```python
from build123d import *

# Parameters (mm, degrees)
SKETCH1_W                   = 77
SKETCH1_H                   = 24
BOSS_EXTRUDE1_DEPTH         = 6
CUT_EXTRUDE1_REACH          = 8
TAP_DRILL_FOR_M3_TAP1_D     = 2.5
TAP_DRILL_FOR_M3_TAP1_DEPTH = 10
TAP_DRILL_FOR_M3_TAP1_TIP   = 0.751075774
TAP_DRILL_FOR_M3_TAP2_D     = 2.5
TAP_DRILL_FOR_M3_TAP2_DEPTH = 10
TAP_DRILL_FOR_M3_TAP2_TIP   = 0.751075774
FILLET1_R                   = 1.5


with BuildPart() as part:
    # Sketch1 → Boss-Extrude1 (new body)
    with BuildSketch(Plane(origin=(0, 0, 0), x_dir=(1, 0, 0), z_dir=(0, 1, 0))):
        with Locations((38.5, 12)):
            Rectangle(SKETCH1_W, SKETCH1_H)
    extrude(amount=BOSS_EXTRUDE1_DEPTH)

    # Sketch2 → Cut-Extrude1 (cut, up to next)
    with BuildSketch(Plane(origin=(0, 6, 0), x_dir=(1, 0, 0), z_dir=(0, 1, 0)), mode=Mode.PRIVATE) as cut_extrude1_sk1:
        Polygon((0, 18), (7, 18), (17.082489299, 11.821127911), (7, 6), (0, 6), align=None)
    cut_extrude1_tool1 = extrude(cut_extrude1_sk1.sketch, amount=-CUT_EXTRUDE1_REACH, mode=Mode.PRIVATE) & part.part
    add(cut_extrude1_tool1.solids().sort_by_distance((6.372388, 6, -11.975038))[0], mode=Mode.SUBTRACT)
    # Sketch2 → Cut-Extrude1 (cut, up to next)
    with BuildSketch(Plane(origin=(0, 6, 0), x_dir=(1, 0, 0), z_dir=(0, 1, 0)), mode=Mode.PRIVATE) as cut_extrude1_sk2:
        Polygon((11.391702814, 20), (65.608297186, 20), (39.5, 4), (37.5, 4), align=None)
    cut_extrude1_tool2 = extrude(cut_extrude1_sk2.sketch, amount=-CUT_EXTRUDE1_REACH, mode=Mode.PRIVATE) & part.part
    add(cut_extrude1_tool2.solids().sort_by_distance((38.5, 6, -14.476924))[0], mode=Mode.SUBTRACT)
    # Sketch2 → Cut-Extrude1 (cut, up to next)
    with BuildSketch(Plane(origin=(0, 6, 0), x_dir=(1, 0, 0), z_dir=(0, 1, 0)), mode=Mode.PRIVATE) as cut_extrude1_sk3:
        Polygon((77, 18), (70, 18), (59.917510701, 11.821127911), (70, 6), (77, 6), align=None)
    cut_extrude1_tool3 = extrude(cut_extrude1_sk3.sketch, amount=-CUT_EXTRUDE1_REACH, mode=Mode.PRIVATE) & part.part
    add(cut_extrude1_tool3.solids().sort_by_distance((70.627612, 6, -11.975038))[0], mode=Mode.SUBTRACT)
    # Sketch2 → Cut-Extrude1 (cut, up to next)
    with BuildSketch(Plane(origin=(0, 6, 0), x_dir=(1, 0, 0), z_dir=(0, 1, 0)), mode=Mode.PRIVATE) as cut_extrude1_sk4:
        Polygon((20.963241239, 9.442878935), (11.535898385, 4), (29.844760038, 4), align=None)
    cut_extrude1_tool4 = extrude(cut_extrude1_sk4.sketch, amount=-CUT_EXTRUDE1_REACH, mode=Mode.PRIVATE) & part.part
    add(cut_extrude1_tool4.solids().sort_by_distance((20.7813, 6, -5.814293))[0], mode=Mode.SUBTRACT)
    # Sketch2 → Cut-Extrude1 (cut, up to next)
    with BuildSketch(Plane(origin=(0, 6, 0), x_dir=(1, 0, 0), z_dir=(0, 1, 0)), mode=Mode.PRIVATE) as cut_extrude1_sk5:
        Polygon((47.155239962, 4), (56.036758761, 9.442878935), (65.464101615, 4), align=None)
    cut_extrude1_tool5 = extrude(cut_extrude1_sk5.sketch, amount=-CUT_EXTRUDE1_REACH, mode=Mode.PRIVATE) & part.part
    add(cut_extrude1_tool5.solids().sort_by_distance((56.2187, 6, -5.814293))[0], mode=Mode.SUBTRACT)

    # Tap Drill for M3 Tap1
    with Locations(Plane.ZY):
        with Locations((-21, 3), (-3, 3)):
            Hole(TAP_DRILL_FOR_M3_TAP1_D / 2, depth=TAP_DRILL_FOR_M3_TAP1_DEPTH)
            with Locations((0, 0, -(TAP_DRILL_FOR_M3_TAP1_DEPTH + TAP_DRILL_FOR_M3_TAP1_TIP / 2))):  # 118° drill point
                Cone(0, TAP_DRILL_FOR_M3_TAP1_D / 2, TAP_DRILL_FOR_M3_TAP1_TIP, mode=Mode.SUBTRACT)

    # Tap Drill for M3 Tap2
    with Locations(Plane(origin=(77, 0, 0), x_dir=(0, 0, -1), z_dir=(1, 0, 0))):
        with Locations((3, 3), (21, 3)):
            Hole(TAP_DRILL_FOR_M3_TAP2_D / 2, depth=TAP_DRILL_FOR_M3_TAP2_DEPTH)
            with Locations((0, 0, -(TAP_DRILL_FOR_M3_TAP2_DEPTH + TAP_DRILL_FOR_M3_TAP2_TIP / 2))):  # 118° drill point
                Cone(0, TAP_DRILL_FOR_M3_TAP2_D / 2, TAP_DRILL_FOR_M3_TAP2_TIP, mode=Mode.SUBTRACT)

    # Fillet1
    fillet1_edges = [part.edges().sort_by_distance(p)[0] for p in [
        (7, 3, -18),
        (17.082489299, 3, -11.821127911),
        (7, 3, -6),
        (70, 3, -6),
        (59.917510701, 3, -11.821127911),
        (70, 3, -18),
        (37.5, 3, -4),
        (11.391702814, 3, -20),
        (65.608297186, 3, -20),
        (39.5, 3, -4),
        (20.963241239, 3, -9.442878935),
        (29.844760038, 3, -4),
        (11.535898385, 3, -4),
        (65.464101615, 3, -4),
        (47.155239962, 3, -4),
        (56.036758761, 3, -9.442878935),
    ]]
    fillet(fillet1_edges, radius=FILLET1_R)


solid = part.part
```
The model under review builds one solid part; all positions refer to its coordinate system, in mm. A direction names the side the tool comes from. Round coordinates to 2 decimals unless told otherwise and drop trailing zeros. Order: outer loops, then holes, each group sorted by start corner. A loop starts at its lowest first (then second) coordinate and runs counter-clockwise, first axis right, second up. Notation, with made-up numbers: (2, -3) -> (35, -3) arc R19 ccw to (35, 11) -> close; hole circle Ø5 at (47.5, 20). An arc over 180 degrees is marked (long way). One line per item, written item: value. Start each with the question number.
Q1. Wall thickness on line 1 (Z direction, x = 73.25, y = 3); line 2 (Z direction, x = 16, y = 5); line 3 (Z direction, x = 18.5, y = 4.5): over which ranges is each line inside the solid? List them lowest first.
Q2. Mouldability with a two-part tool opening along Z and no side actions: class faces 4 (the face through (38, 3, 0)), 5 (the face through (77, 2, -22)), 6 (the face through (53.458, 3.042, -7.862)) as released by +Z, released by -Z, zero draft, split by the parting line, or undercut.
Q3. Take a section at B-B (z = -12.25). Write out the cut boundary in (x, y), and give its area (3 significant figures).
Q4. Machinability: for faces 1 (the face through (25.962, 2.958, -5.067)), 2 (the face through (5.07, 3.38, -4.19)), 3 (the face through (74, 3, -6)), which of the approach directions +Z, -Z, +X, -X, +Y, -Y give a long, thin tool a straight path to every point of the face, cutting with its end or side? Answer none if there is none.
Q5. Take a section at D-D (y = 5). Count the separate pieces of the cut face and the enclosed holes in it, and give its area (3 significant figures).
Q6. Clearance check with flat-ended pins moving along their axes: pin 1 Ø1.5 at (y, z) = (3, -3) entering from -X; pin 2 Ø2 at (y, z) = (3, -16) entering from +X. State where each tip first meets the part, or that it passes through.
Q7. Take a section at A-A (x = 72). Write out the cut boundary in (y, z), and give its area (3 significant figures).
Q8. Take a section at C-C (x = 41). Write out the cut boundary in (y, z), and give its area (3 significant figures).
Reported:
1. line 1: z = -24 to -22.25, -19.75 to -18, -6 to -4.25, -1.75 to 0
1. line 2: z = -24 to -19.82, -17.18 to -6.48, -4.52 to 0
1. line 3: z = -24 to -20, -15.64 to -8.02, -4 to 0
2. face 4: released by +Z
2. face 5: zero draft
2. face 6: undercut
3. outline: (15.6, 0) -> (24.04, 0) -> (24.04, 6) -> (15.6, 6) -> close; (52.96, 0) -> (61.4, 0) -> (61.4, 6) -> (52.96, 6) -> close
3. area: 101 mm2
4. face 1: +Y, -Y
4. face 2: -X
4. face 3: +X, +Y, -Y
5. separate pieces: 1
5. enclosed holes: 3
5. area: 1,040 mm2
6. pin 1: stops at x = 10.3
6. pin 2: stops at x = 68.37
7. outline: (0, -24) -> (6, -24) -> (6, -18) -> (0, -18) -> close; (0, -6) -> (6, -6) -> (6, 0) -> (0, 0) -> close; hole circle Ø2.5 at (3, -21); hole circle Ø2.5 at (3, -3)
7. area: 62.2 mm2
8. outline: (0, -24) -> (6, -24) -> (6, -20) -> (0, -20) -> close; (0, -4.92) -> (6, -4.92) -> (6, 0) -> (0, 0) -> close
8. area: 53.5 mm2
